Answer from the drawing. Dimensions are ordinates in mm from the lowest x, y and z of the part. A direction names the side the tool comes from. Give positions to 0.01 mm unless a question says otherwise; leave off trailing zeros. Loops run counter-clockwise (first coordinate to the right, second up) from the corner with the lowest first, then second, coordinate; pieces in that order, holes last. Notation, with made-up numbers: (-7, -10.5) -> (9, -10.5) arc R30 ccw to (9, 25.5) -> close; hole circle Ø2 at (57.5, 52). An arc over 180 degrees is marked (long way). Answer as CSV lines item,"result". Start each with the question number.
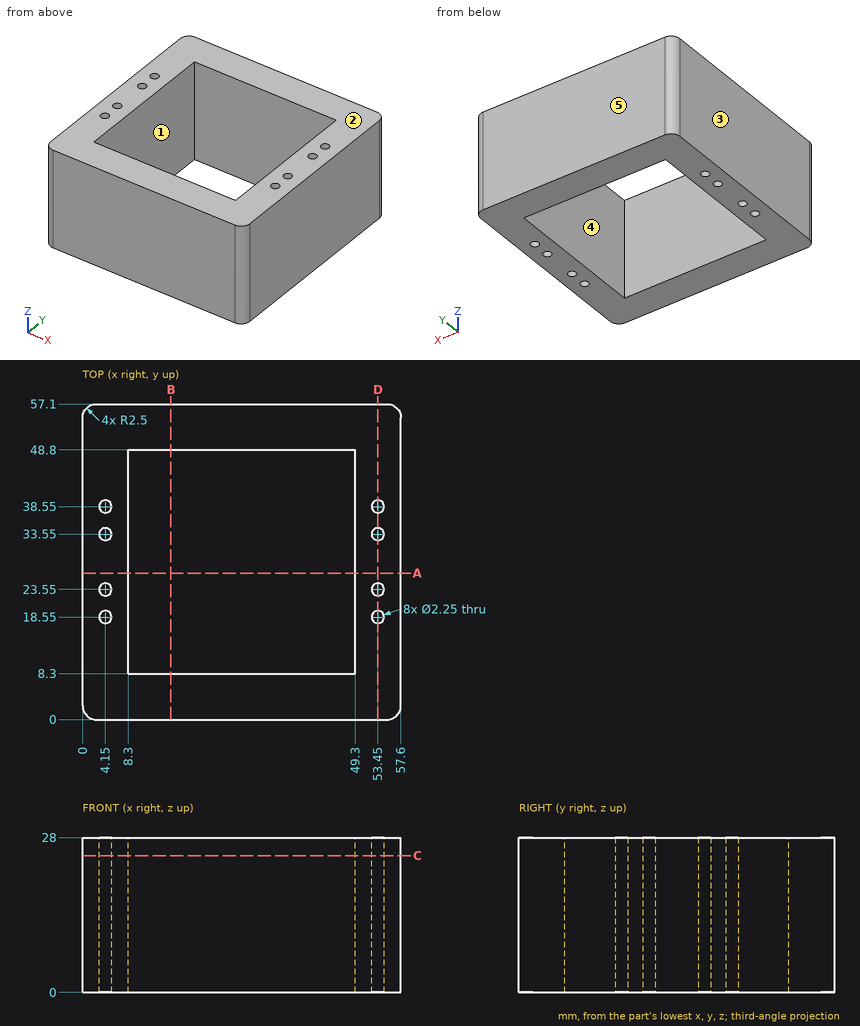
(1) This flat-tipped pin is pushed along its axis until it touches: P1, Ø2, axis at x = 53.45, y = 38.55, coming from the -Z side. Where does it stop, or does it pass through?
(2) Find section D-D on x = 53.45. Write down the section's boundary in (y, z) (3 decimals).
(3) Find section A-A on y = 26.5. Write down the section's boundary in (x, z).
(4) The mould has two halves that part along X. Classify the marked faces 3, 4 and 5: pulls with the +X half, pulls with the -X half, needs draft (parallel to the pull), parting line crosses it, or undercut.
(5) A tool of negligible diameter and unlimited length cuts with its end or side. For the marked faces 1 and 2, from which of +Z, -Z, +X, -X, +Y, -Y can it reach the whole face along a straight path? Write none if from no direction.
(6) Find section C-C on z = 24.75. Give the number of separate pieces and of enclosed holes in the cut face, then the cut area to 3 significant figures.
(7) Find section B-B on x = 16. Write down the section's boundary in (y, z).
(8) Find the intervals of material crossed by line 1 along Y through (x, z) = (53.45, 21) (3 decimals); line 2 along X through (y, z) = (18.5, 6.75); line 3 along X through (y, z) = (40, 12), in increasing order. Write a range as from..to.
Answer block:
1,P1,"passes through"
2,outline,"(0, 0) -> (17.425, 0) -> (17.425, 28) -> (0, 28) -> close; (19.675, 0) -> (22.425, 0) -> (22.425, 28) -> (19.675, 28) -> close; (24.675, 0) -> (32.425, 0) -> (32.425, 28) -> (24.675, 28) -> close; (34.675, 0) -> (37.425, 0) -> (37.425, 28) -> (34.675, 28) -> close; (39.675, 0) -> (57.1, 0) -> (57.1, 28) -> (39.675, 28) -> close"
3,outline,"(0, 0) -> (8.3, 0) -> (8.3, 28) -> (0, 28) -> close; (49.3, 0) -> (57.6, 0) -> (57.6, 28) -> (49.3, 28) -> close"
4,face 3,"pulls with the -X half"
4,face 4,"undercut"
4,face 5,"needs draft"
5,face 1,"+Z, -Z"
5,face 2,"+Z, +X, -X, +Y, -Y"
6,separate pieces,"1"
6,enclosed holes,"9"
6,area,"1,590 mm2"
7,outline,"(0, 0) -> (8.3, 0) -> (8.3, 28) -> (0, 28) -> close; (48.8, 0) -> (57.1, 0) -> (57.1, 28) -> (48.8, 28) -> close"
8,line 1,"y = 0..17.425, 19.675..22.425, 24.675..32.425, 34.675..37.425, 39.675..57.1"
8,line 2,"x = 0..3.03, 5.27..8.3, 49.3..52.33, 54.57..57.6"
8,line 3,"x = 0..8.3, 49.3..57.6"
